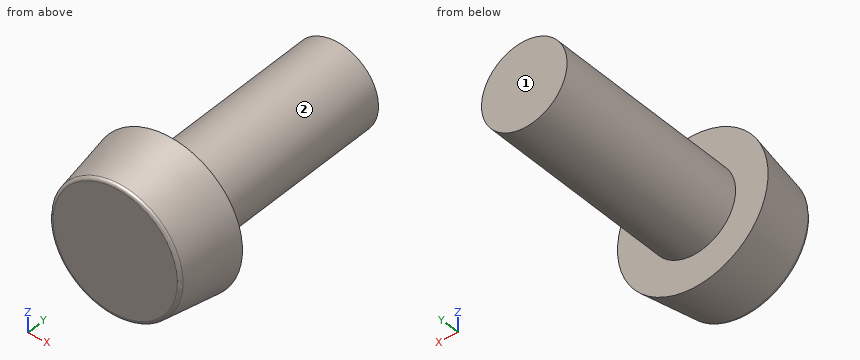
```python
from build123d import *

# Parameters (mm, degrees)
ESQUISSE1_R        = 2.2
BOSS_EXTRU_1_DEPTH = 1.85
ESQUISSE2_R        = 1.25
BOSS_EXTRU_2_DEPTH = 6
CHANFREIN1_SIZE    = 1.85
CHANFREIN1_SIZE_2  = 0.3
CONG_1_R           = 0.1


with BuildPart() as part:
    # Esquisse1 → Boss.-Extru.1 (new body)
    with BuildSketch(Plane(origin=(0, 0, 0), x_dir=(1, 0, 0), z_dir=(0, 1, 0))):
        with Locations(Location((0, 0, 0), (0, 0, 270))):
            Circle(ESQUISSE1_R)
    extrude(amount=BOSS_EXTRU_1_DEPTH)

    # Esquisse2 → Boss.-Extru.2 (add)
    with BuildSketch(Plane(origin=(0, 1.85, 0), x_dir=(1, 0, 0), z_dir=(0, 1, 0))):
        with Locations(Location((0, 0, 0), (0, 0, 270))):
            Circle(ESQUISSE2_R)
    extrude(amount=BOSS_EXTRU_2_DEPTH)

    # Chanfrein1
    # the kernel refuses this chamfer: 1.85, 0.3 mm, written as the material it takes off along each edge
    with BuildSketch(Plane(origin=(0, 0, 0), x_dir=(0, 0, 1), z_dir=(-1, 0, 0))) as chanfrein1_piece_1:
        Polygon((2.2, CHANFREIN1_SIZE), (2.2 - CHANFREIN1_SIZE_2, 0), (2.2, 0), align=None)
    revolve(axis=Axis((0, 0, 0), (0, 1, 0)), mode=Mode.SUBTRACT)

    # Congé1
    cong_1_edges = [part.edges().sort_by_distance(p)[0] for p in [
        (0, 0, -1.9),
    ]]
    fillet(cong_1_edges, radius=CONG_1_R)


solid = part.part
```
Geometry check sheet. Reference: the model listing, model coordinates, mm. Face numbers are marked on the shaded views. A direction names the side the tool comes from. Coordinates: 2 decimals unless noted, no trailing zeros. Order: outer loops, then holes, each group sorted by start corner. A loop starts at its lowest first (then second) coordinate and runs counter-clockwise, first axis right, second up. Notation, with made-up numbers: (37.25, 72.5) - (93.25, 72.5) arc R12 cw to (93.25, 91.5) - close; hole circle Ø6 at (59, 87). An arc over 180 degrees is marked (long way). Answer as a JSON object with one key per item and string values. Group by question number.
Item 1: Scan lines: probe 1 along Y at (x, z) = (1.2, 0.5); probe 2 along Z at (x, y) = (0.55, 2.25); probe 3 along X at (y, z) = (1.75, -1). Record each from-to range of solid material in increasing order.
Item 2: Sectioned sample at A-A, the plane x = 0. Record the cut outline in (y, z), and give its area (3 significant figures).
Item 3: Sectioned sample at B-B, the plane z = 0. Record the cut outline in (x, y).
Item 4: Sectioned sample at C-C, the plane y = 6. Record the cut outline in (x, z), and give its area (3 significant figures).
Item 5: Sectioned sample at D-D, the plane y = 1.5. Record the cut outline in (x, z).
Item 6: Tool access check on the marked faces 1 and 2. Record the directions out of +Z, -Z, +X, -X, +Y, -Y that give a thin tool (end or side, any length) a straight path to the whole face; none if there is none.
Resolved:
{
 "1": {"probe 1": "0 to 1.85", "probe 2": "-1.12 to 1.12", "probe 3": "-1.94 to 1.94"},
 "2": {"outline": "(0, -1.81) arc R0.1 ccw to (0.08, -1.91) - (1.85, -2.2) - (1.85, -1.25) - (7.85, -1.25) - (7.85, 1.25) - (1.85, 1.25) - (1.85, 2.2) - (0.08, 1.91) arc R0.1 ccw to (0, 1.81) - close", "area": "22.6 mm^2"},
 "3": {"outline": "(-2.2, 1.85) - (-1.91, 0.08) arc R0.1 ccw to (-1.81, 0) - (1.81, 0) arc R0.1 ccw to (1.91, 0.08) - (2.2, 1.85) - (1.25, 1.85) - (1.25, 7.85) - (-1.25, 7.85) - (-1.25, 1.85) - close"},
 "4": {"outline": "circle Ø2.5 at (0, 0)", "area": "4.91 mm^2"},
 "5": {"outline": "circle Ø4.29 at (0, 0)"},
 "6": {"face 1": "+Z, -Z, +X, -X, +Y", "face 2": "+Y"}
}
